from build123d import *

# Parameters (mm, degrees)
SKETCH6_R           = 24
BOSS_EXTRUDE1_DEPTH = 6
SKETCH8_R           = 1.55
SKETCH8_R_2         = 2.2
CUT_EXTRUDE6_DEPTH  = 6
SKETCH11_R          = 4.2
CUT_EXTRUDE7_DEPTH  = 3.5
SKETCH12_R          = 3.5
CUT_EXTRUDE8_DEPTH  = 3


with BuildPart() as part:
    # Sketch6 → Boss-Extrude1 (new body)
    with BuildSketch(Plane.XY):
        Circle(SKETCH6_R)
    extrude(amount=BOSS_EXTRUDE1_DEPTH)

    # Sketch8 → Cut-Extrude6 (cut)
    with BuildSketch(Plane(origin=(0, 0, 0), x_dir=(-1, 0, 0), z_dir=(0, 0, -1))):
        with Locations((0, 20)):
            Circle(SKETCH8_R)
        with Locations((14.142135624, 14.142135624)):
            Circle(SKETCH8_R)
        with Locations((20, 0)):
            Circle(SKETCH8_R)
        with Locations((14.142135624, -14.142135624)):
            Circle(SKETCH8_R)
        with Locations((0, -20)):
            Circle(SKETCH8_R)
        with Locations((-14.142135624, -14.142135624)):
            Circle(SKETCH8_R)
        with Locations((-20, 0)):
            Circle(SKETCH8_R)
        with Locations((-14.142135624, 14.142135624)):
            Circle(SKETCH8_R)
        with Locations((11.08655439, 4.592201188)):
            Circle(SKETCH8_R_2)
        with Locations((4.592201188, -11.08655439)):
            Circle(SKETCH8_R_2)
        with Locations((-11.08655439, -4.592201188)):
            Circle(SKETCH8_R_2)
        with Locations((-4.592201188, 11.08655439)):
            Circle(SKETCH8_R_2)
    extrude(amount=-CUT_EXTRUDE6_DEPTH, mode=Mode.SUBTRACT)

    # Sketch11 → Cut-Extrude7 (cut)
    with BuildSketch(Plane.XY.offset(6)):
        with Locations((-11.08655439, 4.592201188)):
            Circle(SKETCH11_R)
        with Locations((4.592201188, 11.08655439)):
            Circle(SKETCH11_R)
        with Locations((11.08655439, -4.592201188)):
            Circle(SKETCH11_R)
        with Locations((-4.592201188, -11.08655439)):
            Circle(SKETCH11_R)
    extrude(amount=-CUT_EXTRUDE7_DEPTH, mode=Mode.SUBTRACT)

    # Sketch12 → Cut-Extrude8 (cut)
    with BuildSketch(Plane(origin=(0, 0, 0), x_dir=(-1, 0, 0), z_dir=(0, 0, -1))):
        with Locations((0, 20)):
            Circle(SKETCH12_R)
        with Locations((14.142135624, 14.142135624)):
            Circle(SKETCH12_R)
        with Locations((20, 0)):
            Circle(SKETCH12_R)
        with Locations((14.142135624, -14.142135624)):
            Circle(SKETCH12_R)
        with Locations((0, -20)):
            Circle(SKETCH12_R)
        with Locations((-14.142135624, -14.142135624)):
            Circle(SKETCH12_R)
        with Locations((-20, 0)):
            Circle(SKETCH12_R)
        with Locations((-14.142135624, 14.142135624)):
            Circle(SKETCH12_R)
    extrude(amount=-CUT_EXTRUDE8_DEPTH, mode=Mode.SUBTRACT)


solid = part.part
Geometry check sheet. Reference: the model listing, model coordinates, mm. A direction names the side the tool comes from. Give positions to 0.01 mm unless a question says otherwise; leave off trailing zeros. Order: outer loops, then holes, each group sorted by start corner. A loop starts at its lowest first (then second) coordinate and runs counter-clockwise, first axis right, second up. Notation, with made-up numbers: (-39.5, -31) - (15.5, -31) arc R25 cw to (15.5, 4) - close; hole circle Ø7 at (65.25, 41.5). An arc over 180 degrees is marked (long way). Answer as a JSON object with one key per item and string values.
(1) Cross-section at B-B (z = 5.45). State how many separate pieces and enclosed holes the cut face has, then the cut area to 3 significant figures.
Report:
{"separate pieces": "1", "enclosed holes": "12", "area": "1,530 mm^2"}
(2) Material ranges on line 1 (Y direction, x = 0, z = 5.65); line 2 (Y direction, x = 13.5, z = 2.35); line 3 (X direction, y = -3, z = 0.85), recorded low to high.
Report:
{"line 1": "-24 to -21.55, -18.45 to 18.45, 21.55 to 24", "line 2": "-19.84 to -17.58, -10.7 to 10.7, 17.58 to 19.84", "line 3": "-23.81 to -21.8, -18.2 to 9.57, 12.6 to 18.2, 21.8 to 23.81"}
(3) Cross-section at A-A (x = 20). Record the cut outline in (y, z).
Report:
{"outline": "(-13.27, 0) - (-3.5, 0) - (-3.5, 3) - (-1.55, 3) - (-1.55, 6) - (-13.27, 6) - close; (1.55, 3) - (3.5, 3) - (3.5, 0) - (13.27, 0) - (13.27, 6) - (1.55, 6) - close"}
(4) Draft check along X on faces 4 (the flat face through (-9, 3, 2.5)), 5 (the flat face through (0, 0, 6)), 6 (the cylindrical face through (-23.977, 1.055, 2.958)). Enter one of: released by +X, released by -X, zero draft, split by the parting line, or undercut.
Report:
{"face 4": "undercut", "face 5": "zero draft", "face 6": "split by the parting line"}
(5) Tool access check on faces 1 (the cylindrical face through (9.9, -2.74, 1.23)), 2 (the cylindrical face through (12.53, -17.25, 1.48)), 3 (the cylindrical face through (-2.65, -14.81, 4.27)). Record the directions out of +Z, -Z, +X, -X, +Y, -Y that give a thin tool (end or side, any length) a straight path to the whole face; none if there is none.
Report:
{"face 1": "+Z, -Z", "face 2": "-Z", "face 3": "+Z"}
(6) Depth check by flat-ended pin: pin 1 Ø3.5 at (x, y) = (20, 0) entering from +Z; pin 2 Ø2 at (x, y) = (15.5, -13.5) entering from -Z; pin 3 Ø3 at (x, z) = (-13, 5) entering from -Y; pin 4 Ø2.5 at (x, y) = (4.5, 10) entering from +Z. Enter the tip coordinate at first touch or a pass-through.
Report:
{"pin 1": "z = 6", "pin 2": "z = 3", "pin 3": "y = -21.07", "pin 4": "z = 2.5"}
(7) Cross-section at D-D (x = 7.5). Record the cut outline in (y, z), then the cut area to 3 significant figures.
Report:
{"outline": "(-22.8, 0) - (22.8, 0) - (22.8, 6) - (14.12, 6) - (14.12, 2.5) - (8.06, 2.5) - (8.06, 6) - (-2.41, 6) - (-2.41, 2.5) - (-6.78, 2.5) - (-6.78, 6) - (-22.8, 6) - close", "area": "237 mm^2"}
